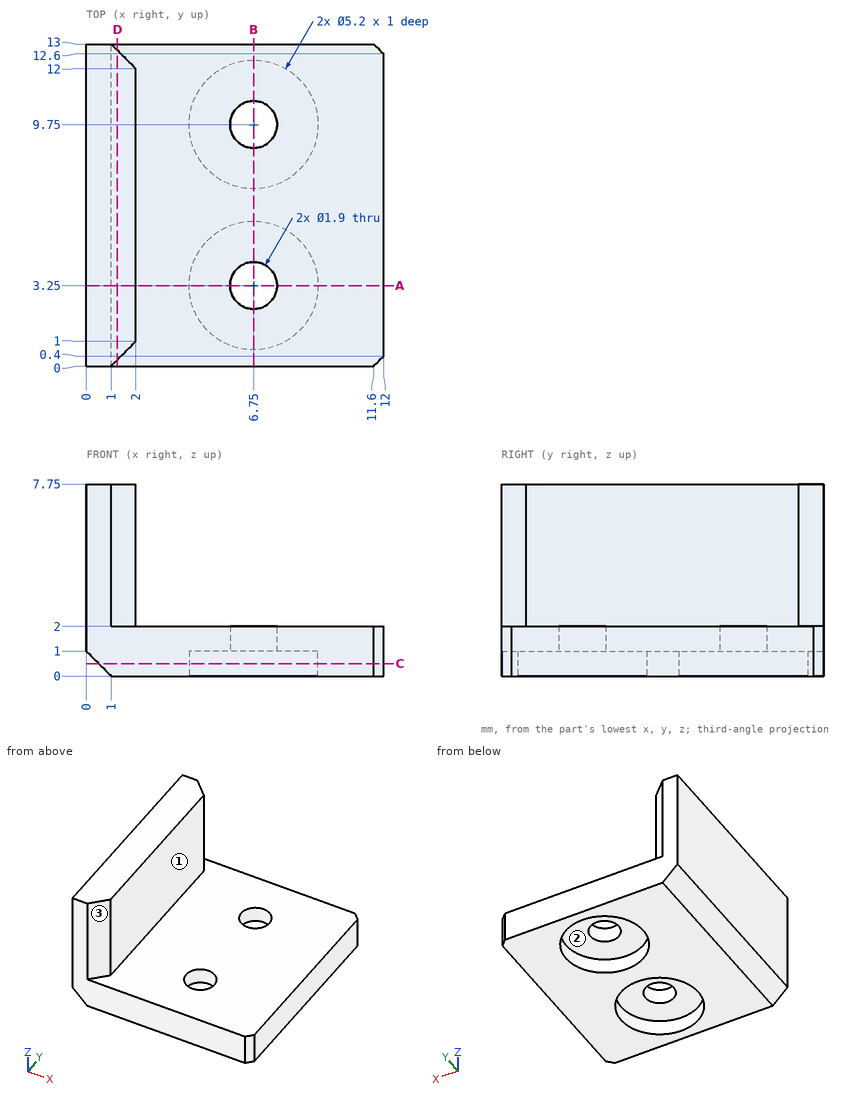
For this review, use the dimensioned drawing (mm, ordinates from the lowest corner) and the shaded views. A direction names the side the tool comes from. Give positions to 0.01 mm unless a question says otherwise; leave off trailing zeros. Write each loop counter-clockwise with the first axis right and the second up, starting at its lowest first coordinate (ties: lowest second). Pieces come first, ordered by that corner, then holes. Notation, with made-up numbers: M 38.25,46 L 84.25,46 A19 cw 84.25,62 Z; hole C -5,40.5 d6. An arc over 180 degrees is marked long. Write item = value, one per line. Start each with the question number.
Q1. We need section A-A (y = 3.25). State the section outline as (x, z) points.
Q2. Machinability: for the marked faces 1, 2 and 3, which of the approach directions +Z, -Z, +X, -X, +Y, -Y give a long, thin tool a straight path to every point of the face, cutting with its end or side? Answer none if there is none.
Q3. We need section B-B (x = 6.75). State the section outline as (y, z) points.
Q4. We need section C-C (z = 0.5). State the section outline as (x, y) points, plus the area to 3 significant figures.
Q5. Clearance check with flat-ended pins moving along their axes: pin 1 (7 mm diameter, centred on x = 6.75, y = 9.75, fed in from +Z); pin 2 (1.1 mm diameter, centred on x = 6.75, y = 9.75, fed in from +Z). State where each tip first meets the part, or that it passes through.
Q6. For line 1 (Y direction, x = 6.75, z = 0.7); line 2 (Y direction, x = 6.75, z = 1.5); line 3 (X direction, y = 9.75, z = 1.7), list the stretches that pass through material, from the lowest coordinate up.
Q7. We need section D-D (x = 1.25). State the section outline as (y, z) points, plus the area to 3 significant figures.
Result set:
q1.outline = M 0,1 L 1,0 L 4.15,0 L 4.15,1 L 5.8,1 L 5.8,2 L 2,2 L 2,7.75 L 0,7.75 Z; M 7.7,1 L 9.35,1 L 9.35,0 L 12,0 L 12,2 L 7.7,2 Z
q2.face_1 = +Z, +X, +Y, -Y
q2.face_2 = -Z
q2.face_3 = +Z, +X, -Y
q3.outline = M 0,0 L 0.65,0 L 0.65,1 L 2.3,1 L 2.3,2 L 0,2 Z; M 4.2,1 L 5.85,1 L 5.85,0 L 7.15,0 L 7.15,1 L 8.8,1 L 8.8,2 L 4.2,2 Z; M 10.7,1 L 12.35,1 L 12.35,0 L 13,0 L 13,2 L 10.7,2 Z
q4.outline = M 0.5,0 L 11.6,0 L 12,0.4 L 12,12.6 L 11.6,13 L 0.5,13 Z; hole C 6.75,3.25 d5.2; hole C 6.75,9.75 d5.2
q4.area = 107 mm2
q5.pin_1 = 2
q5.pin_2 = through
q6.line_1 = 0 to 0.65, 5.85 to 7.15, 12.35 to 13
q6.line_2 = 0 to 2.3, 4.2 to 8.8, 10.7 to 13
q6.line_3 = 0 to 5.8, 7.7 to 12
q7.outline = M 0,0 L 13,0 L 13,2 L 12.75,2 L 12.75,7.75 L 0.25,7.75 L 0.25,2 L 0,2 Z
q7.area = 97.9 mm2
